The listing builds one solid part. Answer for the finished solid, in the listing's coordinates (mm). Face numbers are marked on the shaded views. A direction names the side the tool comes from. Round coordinates to 2 decimals unless told otherwise and drop trailing zeros. Loops run counter-clockwise (first coordinate to the right, second up) from the corner with the lowest first, then second, coordinate; pieces in that order, holes last. Notation, with made-up numbers: (10.5, 30) -> (20.5, 30) arc R30 ccw to (20.5, 54) -> close; hole circle Ø9 at (-17, 11). An arc over 180 degrees is marked (long way). Use a Markdown table: item, result. Add a question column.
Q1. Given pin 1 Ø1 at (x, z) = (-1, 1.5) entering from +Y; pin 2 Ø1 at (x, z) = (-2, 1) entering from -Y; pin 3 Ø1.5 at (x, z) = (-2, -1.5) entering from +Y, each flat-ended and moving along its own axis, determine where each tip first touches the part or whether it passes through.
Q2. Section D-D on x = 1.65 is taken. Give the vertices of the cut face in (y, z) (3 decimals).
Q3. For a pull along Y with two mould halves and no side action, classify the marked faces 3, 4 and 5 as released by +Y, released by -Y, zero draft, split by the parting line, or undercut.
Q4. Which of the six approach directions +Z, -Z, +X, -X, +Y, -Y give full straight-line access (tool end or side, diameter ignored) to the marked faces 1 and 2?
Q5. Consider line 1 (Z direction, x = -0.9, y = 0) (3 decimals); line 2 (X direction, y = 2, z = 2.5); line 3 (Y direction, x = 2.65, z = -1.25). Determine where each line is inside the solid, lowest interval first.
Q6. Section C-C on x = -1.55 is taken. Give the vertices of the cut face in (y, z) (3 decimals), then the cut area to 3 significant figures.
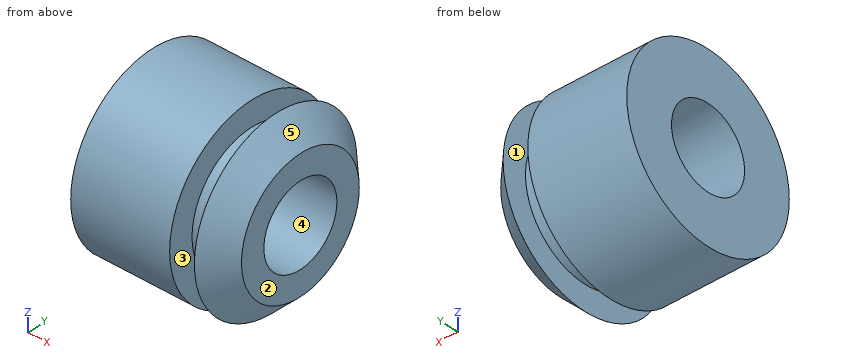
Autodesk Inventor part; units mm, degrees
ref_plane "作業平面1" through (2, 0, 0) normal (1, 0, 0) x (0, 0, -1)
ref_plane "YZ Plane" through (0, 0, 0) normal (1, 0, 0) x (0, 1, 0)
ref_plane "XZ Plane" through (0, 0, 0) normal (0, 1, 0) x (-1, 0, 0)
sketch "スケッチ1" plane through (0, 0, 0) normal (1, 0, 0) x (0, 1, 0)
  circle A0 centre (0, 0) radius 3.635
  circle A1 centre (0, 0) radius 1.635
  circle A2 centre (0, 0) radius 2.635
  dimension "d0" = 3.27
  dimension "d1" = 2
  dimension "d7" = 1
extrude "押し出し1" add sketch "スケッチ1" along normal mid plane 6 contours A0 | A2
ref_plane "作業平面1" through (2, 0, 0) normal (1, 0, 0) x (0, 0, -1)
extrude "押し出し3" cut sketch "スケッチ1" against normal blind 1 from surface at 2 contours A0
chamfer "面取り3" distance 1 angle 45 1 edges at (3, -3.635, 0)
properties part number "spacer_Φ3.2_1"
Checked values:
| question | item | result |
|---|---|---|
| 1 | pin 1 | stops at y = 3.49 |
| 1 | pin 2 | stops at y = -3.6 |
| 1 | pin 3 | stops at y = 3.56 |
| 2 | outline | circle Ø5.27 at (0, 0); hole circle Ø3.27 at (0, 0) |
| 3 | face 3 | zero draft |
| 3 | face 4 | undercut |
| 3 | face 5 | split by the parting line |
| 4 | face 1 | none |
| 4 | face 2 | +Z, -Z, +X, +Y, -Y |
| 5 | line 1 | z = -3.635 to -1.635, 1.635 to 3.635 |
| 5 | line 2 | x = -3 to 1, 2 to 2.43 |
| 5 | line 3 | y = -2.71 to -1.05, 1.05 to 2.71 |
| 6 | outline | circle Ø7.27 at (0, 0); hole circle Ø3.27 at (0, 0) |
| 6 | area | 33.1 mm2 |
